Verification items for this drawing (mm, ordinates from the low corner). Round coordinates to 2 decimals unless told otherwise and drop trailing zeros. Loops run counter-clockwise (first coordinate to the right, second up) from the corner with the lowest first, then second, coordinate; pieces in that order, holes last. Notation, with made-up numbers: (55, 65.5) - (66, 65.5) arc R21 cw to (66, 100.5) - close; hole circle Ø3 at (1, 50.5). An arc over 180 degrees is marked (long way). Put each result on its own line as item: value.
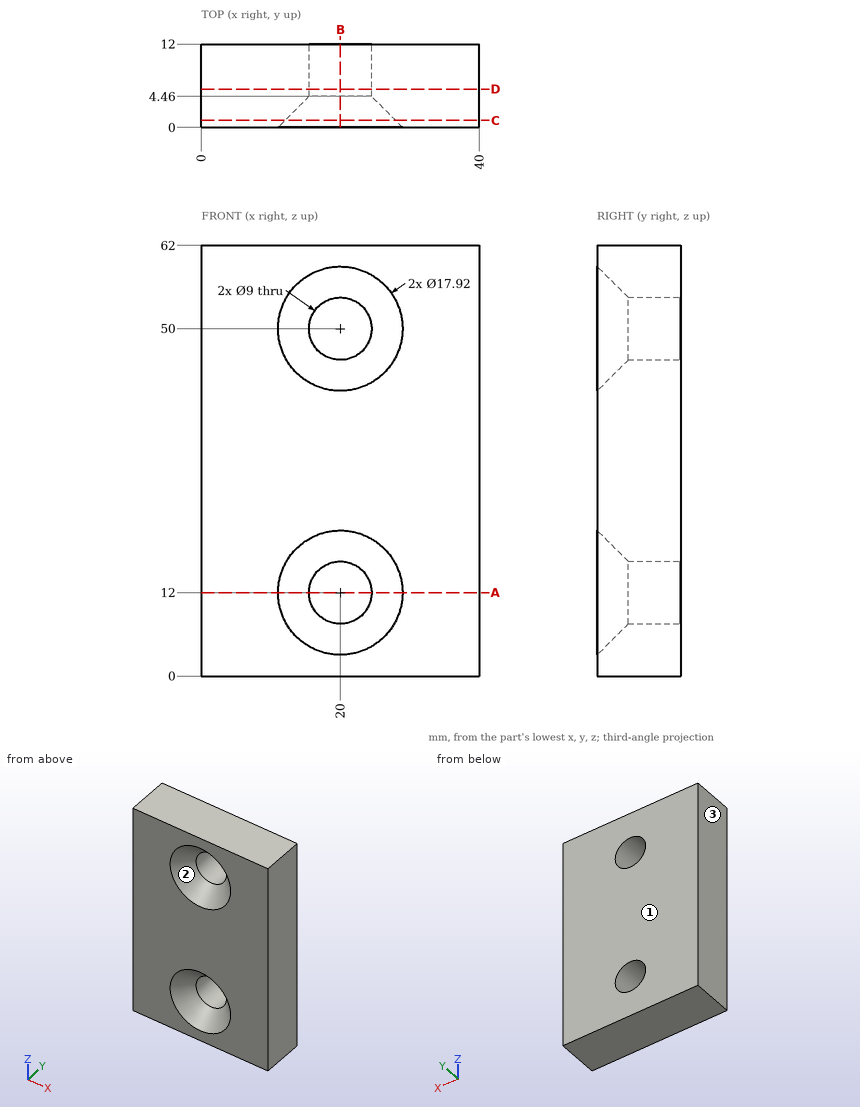
Item 1: Release check for a two-part mould opening along X. For the marked faces 1, 2 and 3 record: +X half, -X half, draft (parallel to the pull), parting line (faces both ways), or undercut.
Filled sheet:
face 1: draft
face 2: undercut
face 3: -X half
Item 2: Section check A-A on z = 12. Enter the section's corners in (x, y).
Filled sheet:
outline: (0, 0) - (11.04, 0) - (15.5, 4.46) - (15.5, 12) - (0, 12) - close; (24.5, 4.46) - (28.96, 0) - (40, 0) - (40, 12) - (24.5, 12) - close
Item 3: Go/stop test with flat-tipped pins: pin 1 (6 mm diameter, centred on y = 1.5, z = 22.5, fed in from -X); pin 2 (1 mm diameter, centred on x = 19, z = 43.5, fed in from -Y). Record where each tip stops, or that it passes through.
Filled sheet:
pin 1: x = 0
pin 2: y = 1.88
Item 4: Section check B-B on x = 20. Enter the section's corners in (y, z), then the cut area to 3 significant figures.
Filled sheet:
outline: (0, 0) - (12, 0) - (12, 7.5) - (4.46, 7.5) - (0, 3.04) - close; (0, 20.96) - (4.46, 16.5) - (12, 16.5) - (12, 45.5) - (4.46, 45.5) - (0, 41.04) - close; (0, 58.96) - (4.46, 54.5) - (12, 54.5) - (12, 62) - (0, 62) - close
area: 488 mm²
Item 5: Section check C-C on y = 1. Enter the section's corners in (x, z).
Filled sheet:
outline: (0, 0) - (40, 0) - (40, 62) - (0, 62) - close; hole circle Ø15.92 at (20, 12); hole circle Ø15.92 at (20, 50)
Item 6: Thickness scan on line 1 (Z direction, x = 20, y = 6.5); line 2 (X direction, y = 8.25, z = 50); line 3 (Z direction, x = 19, y = 11.25). Record the ranges inside material, lowest first. Write a range as from..to.
Filled sheet:
line 1: 0..7.5, 16.5..45.5, 54.5..62
line 2: 0..15.5, 24.5..40
line 3: 0..7.61, 16.39..45.61, 54.39..62
Item 7: Section check D-D on y = 5.5. Enter the section's corners in (x, z).
Filled sheet:
outline: (0, 0) - (40, 0) - (40, 62) - (0, 62) - close; hole circle Ø9 at (20, 12); hole circle Ø9 at (20, 50)
